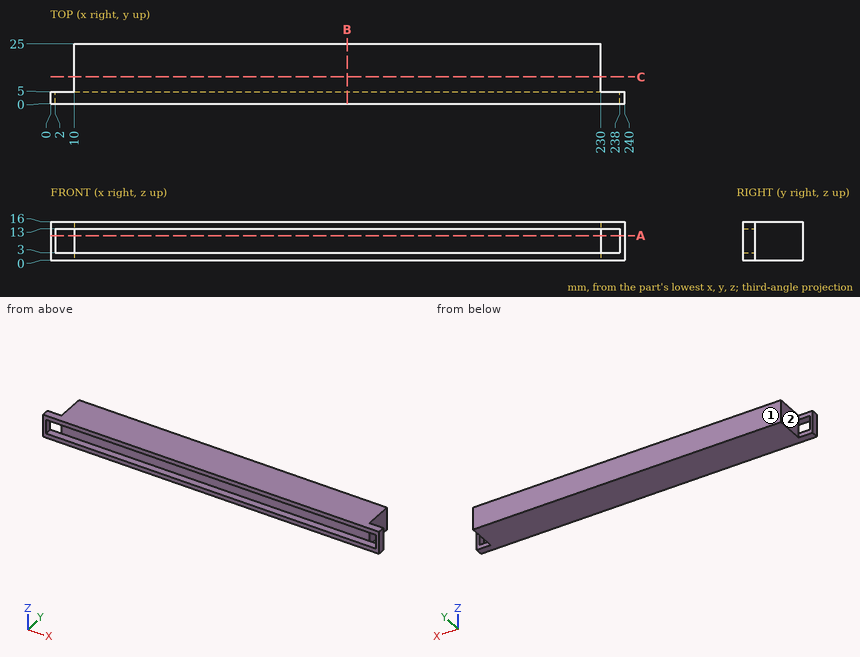
Verification items for this drawing (mm, ordinates from the low corner). A direction names the side the tool comes from. Coordinates: 2 decimals unless noted, no trailing zeros. Order: outer loops, then holes, each group sorted by start corner. A loop starts at its lowest first (then second) coordinate and runs counter-clockwise, first axis right, second up. Notation, with made-up numbers: M 33.5,9.5 L 81.5,9.5 A24 cw 81.5,38.5 Z; hole C -12.5,9.5 d7. An arc over 180 degrees is marked long. One line per item, written item: value. Start each with the question number.
Item 1: Thickness scan on probe 1 along Z at (x, y) = (69, 3); probe 2 along Y at (x, z) = (212, 4.5); probe 3 along X at (y, z) = (9.75, 1.75). Record the ranges inside material, lowest first.
Item 2: Sectioned sample at C-C on y = 11.25. Record the cut outline in (x, z), then the cut area to 3 significant figures.
Item 3: Sectioned sample at A-A on z = 10.25. Record the cut outline in (x, y).
Item 4: Sectioned sample at B-B on x = 124. Record the cut outline in (y, z), then the cut area to 3 significant figures.
Item 5: Access from +Z, -Z, +X, -X, +Y, -Y to the whole of each face (thin tool, end or side, straight path). Record for the marked faces 1 and 2.
Item 6: Depth check by flat-ended pin: P1, Ø4, axis at x = 122.5, z = 7, coming from the -Y side; P2, Ø1, axis at y = 19, z = 3, coming from the +X side; P3, Ø1.5, axis at y = 18, z = 8, coming from the -X side. Enter the tip coordinate at first touch or a pass-through.
Calculated:
1. probe 1: 0 to 3, 13 to 16
1. probe 2: 5 to 25
1. probe 3: 10 to 230
2. outline: M 10,0 L 230,0 L 230,16 L 10,16 Z
2. area: 3,520 mm^2
3. outline: M 0,0 L 2,0 L 2,5 L 0,5 Z; M 10,5 L 230,5 L 230,25 L 10,25 Z; M 238,0 L 240,0 L 240,5 L 238,5 Z
4. outline: M 0,0 L 25,0 L 25,16 L 0,16 L 0,13 L 5,13 L 5,3 L 0,3 Z
4. area: 350 mm^2
5. face 1: +Z, -Z, +X, -X, +Y
5. face 2: +Z, -Z, -X, +Y
6. P1: y = 5
6. P2: x = 230
6. P3: x = 10
